Read the model definition and answer for the solid it produces. Units are mm, in the model's axes. Give positions to 0.01 mm unless a question says otherwise; leave off trailing zeros. Write each loop counter-clockwise with the first axis right and the second up, starting at its lowest first coordinate (ties: lowest second). Pieces come first, ordered by that corner, then holes. Notation, with made-up numbers: (68.25, 56) -> (123.25, 56) arc R21 cw to (123.25, 80) -> close; hole circle Ø3 at (-22.5, -26). An arc over 180 degrees is marked (long way). Use a Markdown table: item, result.
from build123d import *

# Parameters (mm, degrees)
SKETCH1_W           = 25.2
SKETCH1_H           = 34
BOSS_EXTRUDE1_DEPTH = 3.2
CUT_EXTRUDE1_REACH  = 5.2
SKETCH4_R           = 6.86


with BuildPart() as part:
    # Sketch1 → Boss-Extrude1 (new body)
    with BuildSketch(Plane.XY):
        Rectangle(SKETCH1_W, SKETCH1_H)
    extrude(amount=BOSS_EXTRUDE1_DEPTH)

    # Sketch4 → Cut-Extrude1 (cut, up to next)
    with BuildSketch(Plane.XY.offset(3.2), mode=Mode.PRIVATE) as cut_extrude1_sk1:
        with Locations((0, -4.06)):
            Circle(SKETCH4_R)
    cut_extrude1_tool1 = extrude(cut_extrude1_sk1.sketch, amount=-CUT_EXTRUDE1_REACH, mode=Mode.PRIVATE) & part.part
    add(cut_extrude1_tool1.solids().sort_by_distance((0, -4.06, 3.2))[0], mode=Mode.SUBTRACT)


solid = part.part
Item 1: A cutting plane is placed at A-A (y = -4.06). Give the vertices of the cut face in (x, z).
Return value:
| item | result |
|---|---|
| outline | (-12.6, 0) -> (-6.86, 0) -> (-6.86, 3.2) -> (-12.6, 3.2) -> close; (6.86, 0) -> (12.6, 0) -> (12.6, 3.2) -> (6.86, 3.2) -> close |
Item 2: A cutting plane is placed at B-B (x = 0). Give the vertices of the cut face in (y, z), then the cut area to 3 significant figures.
Return value:
| item | result |
|---|---|
| outline | (-17, 0) -> (-10.92, 0) -> (-10.92, 3.2) -> (-17, 3.2) -> close; (2.8, 0) -> (17, 0) -> (17, 3.2) -> (2.8, 3.2) -> close |
| area | 64.9 mm^2 |
Item 3: A cutting plane is placed at C-C (z = 1.6). Give the vertices of the cut face in (x, y), then the cut area to 3 significant figures.
Return value:
| item | result |
|---|---|
| outline | (-12.6, -17) -> (12.6, -17) -> (12.6, 17) -> (-12.6, 17) -> close; hole circle Ø13.72 at (0, -4.06) |
| area | 709 mm^2 |
Item 4: For a pull along X with two mould halves and no side action, classify faces 1 (the face through (6.543, -1.999, 1.622)), 2 (the face through (0, 4, 0)), 3 (the face through (12.6, 0, 2)) as +X half, -X half, draft (parallel to the pull), parting line (faces both ways), or undercut.
Return value:
| item | result |
|---|---|
| face 1 | undercut |
| face 2 | draft |
| face 3 | +X half |
Item 5: This flat-tipped pin is pushed along its axis until it touches: P1, Ø8, axis at x = 0, y = -4.06, coming from the +Z side. Where does it stop, or does it pass through?
Return value:
| item | result |
|---|---|
| P1 | through |
Item 6: Straight lines are drawn through the part: line 1 along Y through (x, z) = (0, 0.8); line 2 along Y through (x, z) = (-2, 2.75); line 3 along X through (y, z) = (-6.5, 2.8). For each, find the intervals that lie inside material, in ascending order. Write a range as [from, to].
Return value:
| item | result |
|---|---|
| line 1 | [-17, -10.92], [2.8, 17] |
| line 2 | [-17, -10.62], [2.5, 17] |
| line 3 | [-12.6, -6.41], [6.41, 12.6] |
